Here's how the part is built. I have some questions about the finished solid (model axes, mm). Face numbers are marked on the shaded views. A direction names the side the tool comes from. Round coordinates to 2 decimals unless told otherwise and drop trailing zeros. Loops run counter-clockwise (first coordinate to the right, second up) from the corner with the lowest first, then second, coordinate; pieces in that order, holes last. Notation, with made-up numbers: M -30.75,69 L -3.75,69 A17 ccw -3.75,94 Z; hole C 30.5,6 d9. An arc over 180 degrees is marked long. Answer as CSV lines item,"result".
```python
from build123d import *

# Parameters (mm, degrees)
F1_DEPTH  = 38.1
F2_W      = 46.7332457192
F2_H      = 0.889
F3_DEPTH  = 20.5994
F5_DEPTH  = 29.21
F7_DEPTH  = 29.21
F8_W      = 22.6521064695
F8_H      = 63.5
F8_W_2    = 36.5288935305
F9_DEPTH  = 2.54
F10_DEPTH = 3
F11_W     = 59.181
F11_H     = 17.9686862156
F12_DEPTH = 69.342
F13_W     = 21.081
F13_H     = 6.35
F14_DEPTH = 3
F15_R     = 1.778
F16_DEPTH = 25.4


with BuildPart() as f1:
    # F0 (on Front) → F1 (new body, symmetric)
    with BuildSketch(Plane.XZ):
        with BuildLine():
            ThreePointArc((9.876787061, -3.4580663421), (15.0923499173, 0.3786818234), (17.081, 6.5405))
            ThreePointArc((17.081, 6.5405), (6.5405, 17.081), (-4, 6.5405))
            ThreePointArc((-4, 6.5405), (-2.0113499173, 0.3786818234), (3.204212939, -3.4580663421))
            Line((3.204212939, -3.4580663421), (9.876787061, -3.4580663421))
        make_face()
        with BuildLine():
            ThreePointArc((6.5405, 0), (1.9156680976, 11.1653319024), (13.081, 6.5405))
            ThreePointArc((13.081, 6.5405), (11.1653319024, 1.9156680976), (6.5405, 0))
        make_face(mode=Mode.SUBTRACT)
        with BuildLine():
            Line((17.081, 0), (17.081, 6.5405))
            ThreePointArc((17.081, 6.5405), (15.0923499173, 0.3786818234), (9.876787061, -3.4580663421))
            Line((9.876787061, -3.4580663421), (17.081, -3.4580663421))
            Line((17.081, -3.4580663421), (17.081, 0))
        make_face()
        with BuildLine():
            ThreePointArc((3.204212939, -3.4580663421), (-2.0113499173, 0.3786818234), (-4, 6.5405))
            Line((-4, 6.5405), (-4, -3.4580663421))
            Line((-4, -3.4580663421), (3.204212939, -3.4580663421))
        make_face()
        with BuildLine():
            ThreePointArc((3.204212939, -3.4580663421), (6.5405, -4), (9.876787061, -3.4580663421))
            Line((9.876787061, -3.4580663421), (3.204212939, -3.4580663421))
        make_face()
    extrude(amount=F1_DEPTH, both=True)

    # F2 (on Top) → F3 (cut)
    with BuildSketch(Plane.XY):
        Rectangle(F2_W, F2_H)
    extrude(amount=F3_DEPTH, mode=Mode.SUBTRACT)

    # F4 (on face) → F5 (cut)
    with BuildSketch(Plane(origin=(0, 38.1, 0), x_dir=(-1, 0, 0), z_dir=(0, 1, 0))):
        with BuildLine():
            ThreePointArc((-17.081, 6.5405), (-7.9427578532, 16.987308755), (3.6269006049, 9.3200872335))
            Line((3.6269006049, 9.3200872335), (4, 28.6066166948))
            Line((4, 28.6066166948), (-17.081, 29.0144302604))
            Line((-17.081, 29.0144302604), (-17.5960424147, 27.9336988817))
            Line((-17.5960424147, 27.9336988817), (-17.081, 6.5405))
        make_face()
        with BuildLine():
            ThreePointArc((-13.081, 6.5405), (-6.5405, 13.081), (0, 6.5405))
            Line((0, 6.5405), (4, 6.5405))
            ThreePointArc((4, 6.5405), (3.906308755, 7.9427578532), (3.6269006049, 9.3200872335))
            ThreePointArc((3.6269006049, 9.3200872335), (-7.9427578532, 16.987308755), (-17.081, 6.5405))
            Line((-17.081, 6.5405), (-13.081, 6.5405))
        make_face()
        with BuildLine():
            Line((-13.081, 6.5405), (0, 6.5405))
            ThreePointArc((0, 6.5405), (-6.5405, 13.081), (-13.081, 6.5405))
        make_face()
    extrude(amount=-F5_DEPTH, mode=Mode.SUBTRACT)

    # F6 (on face) → F7 (cut)
    with BuildSketch(Plane.XZ.offset(38.1)):
        with BuildLine():
            ThreePointArc((0, 6.5405), (6.5405, 13.081), (13.081, 6.5405))
            Line((13.081, 6.5405), (17.081, 6.5405))
            ThreePointArc((17.081, 6.5405), (6.5405, 17.081), (-4, 6.5405))
            Line((-4, 6.5405), (0, 6.5405))
        make_face()
    extrude(amount=-F7_DEPTH, mode=Mode.SUBTRACT)

    # F8 (on face) → F9 (join)
    with BuildSketch(Plane(origin=(0, 0, -3.4580663421), x_dir=(1, 0, 0), z_dir=(0, 0, -1))):
        with Locations((24.8049467652, 0)):
            Rectangle(F8_W, F8_H)
        with Locations((-4.7855532348, 0)):
            Rectangle(F8_W_2, F8_H)
    extrude(amount=-F9_DEPTH)

    # F8 (on face) → F10 (join)
    with BuildSketch(Plane(origin=(0, 0, -3.4580663421), x_dir=(1, 0, 0), z_dir=(0, 0, -1))):
        with Locations((24.8049467652, 0)):
            Rectangle(F8_W, F8_H)
        with Locations((-4.7855532348, 0)):
            Rectangle(F8_W_2, F8_H)
    extrude(amount=F10_DEPTH)

    # F11 (on face) → F12 (cut)
    with BuildSketch(Plane(origin=(0, 0, -6.4580663421), x_dir=(1, 0, 0), z_dir=(0, 0, -1))):
        with Locations((6.5405, -22.7656568922)):
            Rectangle(F11_W, F11_H)
        Polygon((-23.05, -13.7813137844), (-30.0445724279, -13.7813137844), (-30.0445724279, -67.8615421057), (58.1297166646, -67.8615421057), (58.1297166646, -13.7813137844), (36.131, -13.7813137844), (36.131, -31.75), (-23.05, -31.75), align=None)
    extrude(amount=-F12_DEPTH, mode=Mode.SUBTRACT)

    # F13 (on face) → F14 (join, through all)
    with BuildSketch(Plane(origin=(0, 0, -3.4580663421), x_dir=(1, 0, 0), z_dir=(0, 0, -1))):
        with Locations((6.5405, 34.925)):
            Rectangle(F13_W, F13_H)
    extrude(amount=F14_DEPTH)

    # F15 (on face) → F16 (cut)
    with BuildSketch(Plane.XY.offset(-0.9180663421)):
        with Locations((-12.89, -17.8570281714)):
            Circle(F15_R)
        with Locations((25.971, -17.8570281714)):
            Circle(F15_R)
    extrude(amount=-F16_DEPTH, mode=Mode.SUBTRACT)


solid = f1.part
```
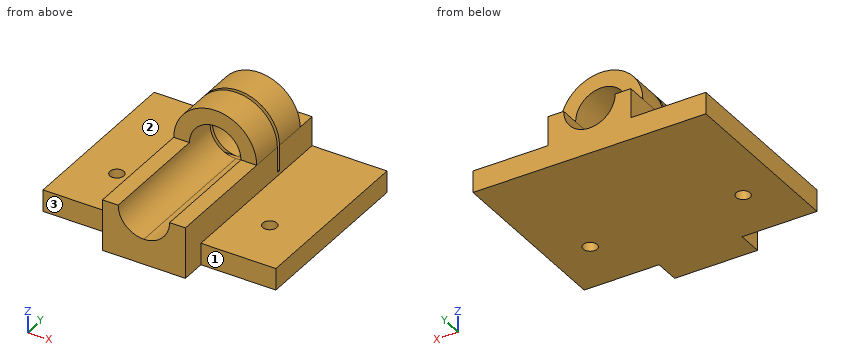
1. If I drill on line 1 (Y direction, x = -12.89, z = -4.15); line 2 (Y direction, x = 16.5, z = 1.75); line 3 (Z direction, x = 18, y = -20), over which ranges is the centre line in solid material (lowest first)? Write a range as [from, to].
Evaluation:
line 1,"y = [-31.75, -19.64], [-16.08, 13.78]"
line 2,"y = [-38.1, -0.44], [0.44, 13.78]"
line 3,"z = [-6.46, -0.92]"
2. For P1, Ø4, axis at x = 15.5, y = -26.5, coming from the +Z side; P2, Ø4.5, axis at x = 22.5, z = -4, coming from the -Y side; P3, Ø3, axis at y = -25.5, z = 2, coming from the -X side, each with a flat end and sliding along its axis, tell me the tip position at first contact or that it passes through.
Evaluation:
P1,"stops at z = 6.54"
P2,"stops at y = -31.75"
P3,"stops at x = -4"
3. I want a section at B-B, the plane y = -1.5. Please give me the cut outline in (x, z).
Evaluation:
outline,"M -23.05,-6.46 L 36.13,-6.46 L 36.13,-0.92 L 17.08,-0.92 L 17.08,6.54 A10.54 ccw -4,6.54 L -4,-0.92 L -23.05,-0.92 Z; hole C 6.54,6.54 d13.08"
4. I want a section at D-D, the plane z = 0.75. Please give me the cut outline in (x, y).
Evaluation:
outline,"M -4,-38.1 L 3.5,-38.1 L 3.5,-0.44 L -4,-0.44 Z; M -4,0.44 L 3.5,0.44 L 3.5,13.78 L -4,13.78 Z; M 9.58,-38.1 L 17.08,-38.1 L 17.08,-0.44 L 9.58,-0.44 Z; M 9.58,0.44 L 17.08,0.44 L 17.08,13.78 L 9.58,13.78 Z"
5. I want a section at C-C, the plane x = 1. Please give me the cut outline in (y, z), and give its area (3 significant figures).
Evaluation:
outline,"M -38.1,-6.46 L 13.78,-6.46 L 13.78,3.06 L 0.44,3.06 L 0.44,0 L -0.44,0 L -0.44,3.06 L -38.1,3.06 Z; M -8.89,10.02 L -0.44,10.02 L -0.44,15.51 L -8.89,15.51 Z; M 0.44,10.02 L 8.89,10.02 L 8.89,15.51 L 0.44,15.51 Z"
area,"584 mm²"
6. I want a section at A-A, the plane x = -12.89. Please give me the cut outline in (y, z), and give its area (3 significant figures).
Evaluation:
outline,"M -31.75,-6.46 L -19.64,-6.46 L -19.64,-0.92 L -31.75,-0.92 Z; M -16.08,-6.46 L 13.78,-6.46 L 13.78,-0.92 L -16.08,-0.92 Z"
area,"233 mm²"
7. Which directions (+Z, -Z, +X, -X, +Y, -Y) give clear straight access to the entire face, cutting with the end or side of a thin tool? Please do the marked faces 1, 2 and 3.
Evaluation:
face 1,"+Z, -Z, +X, -Y"
face 2,"+Z, -X, +Y, -Y"
face 3,"+Z, -Z, -X, -Y"
